The model under review builds one solid part; all positions refer to its coordinate system, in mm. Face numbers are marked on the shaded views. A direction names the side the tool comes from. Coordinates: 2 decimals unless noted, no trailing zeros. Write each loop counter-clockwise with the first axis right and the second up, starting at its lowest first coordinate (ties: lowest second). Pieces come first, ordered by that corner, then holes. Notation, with made-up numbers: (-36.75, 51.25) -> (19.25, 51.25) arc R15 ccw to (19.25, 57.25) -> close; hole circle Ø5 at (-26.75, 48.5). An arc over 180 degrees is marked (long way). Write each question's results on one line, items separated by ' | '.
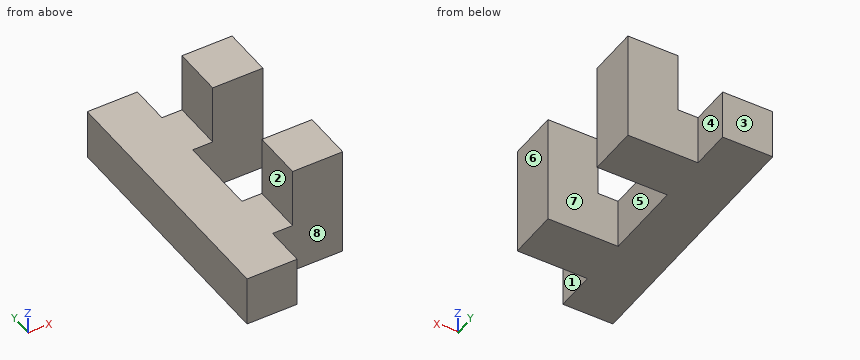
```python
from build123d import *

# Parameters (mm, degrees)
F1_DEPTH = 63.5
F2_W     = 63.5
F2_H     = 63.5
F3_DEPTH = 76.2


with BuildPart() as f1:
    # F0 (on Top) → F1 (new body)
    with BuildSketch(Plane.XY):
        Polygon((63.5, 0), (0, 0), (0, -330.2), (63.5, -330.2), (63.5, -279.4), (152.4, -279.4), (152.4, -215.9), (63.5, -215.9), (63.5, -114.3), (152.4, -114.3), (152.4, -50.8), (63.5, -50.8), align=None)
    extrude(amount=F1_DEPTH)

    # F2 (on face) → F3 (join)
    with BuildSketch(Plane.XY.offset(63.5)):
        with Locations((120.65, -82.55)):
            Rectangle(F2_W, F2_H)
        with Locations((120.65, -247.65)):
            Rectangle(F2_W, F2_H)
    extrude(amount=F3_DEPTH)


solid = f1.part
```
Q1. For line 1 (Y direction, x = 109, z = 94.5); line 2 (X direction, y = -224.5, z = 122); line 3 (X direction, y = -115, z = 59), list the stretches that pass through material, from the lowest coordinate up. Write a range as from..to.
Solution:
line 1: -279.4..-215.9, -114.3..-50.8 | line 2: 88.9..152.4 | line 3: 0..63.5
Q2. Add section B-B (x = 73). Write out the cut boundary in (y, z).
Solution:
outline: (-279.4, 0) -> (-215.9, 0) -> (-215.9, 63.5) -> (-279.4, 63.5) -> close; (-114.3, 0) -> (-50.8, 0) -> (-50.8, 63.5) -> (-114.3, 63.5) -> close
Q3. Machinability: for the marked faces 1, 2, 3, 4 and 5, which of the approach directions +Z, -Z, +X, -X, +Y, -Y give a long, thin tool a straight path to every point of the face, cutting with its end or side? Answer none if there is none.
Solution:
face 1: +Z, -Z, +X, -Y | face 2: +Z, -X, +Y, -Y | face 3: +Z, -Z, +X, -X, +Y | face 4: +Z, -Z, +X, +Y | face 5: +Z, -Z, +X
Q4. Clearance check with flat-ended pins moving along their axes: P1, Ø15, axis at y = -38, z = 18.5, coming from the +X side; P2, Ø3, axis at y = -97, z = 79.5, coming from the -X side; P3, Ø1.5, axis at x = 35.5, y = -232, coming from the +Z side; P4, Ø5, axis at y = -71.5, z = 17.5, coming from the -X side. State where each tip first meets the part, or that it passes through.
Solution:
P1: x = 63.5 | P2: x = 88.9 | P3: z = 63.5 | P4: x = 0
Q5. Draft analysis for pull direction Y (two halves, no side actions). For the marked faces 6, 7 and 8, state which applies: pulls with the +Y half, pulls with the -Y half, needs draft (parallel to the pull), parting line crosses it, or undercut.
Solution:
face 6: needs draft | face 7: undercut | face 8: pulls with the -Y half
Q6. Add section C-C (z = 55.5). Write out the cut boundary in (x, y).
Solution:
outline: (0, -330.2) -> (63.5, -330.2) -> (63.5, -279.4) -> (152.4, -279.4) -> (152.4, -215.9) -> (63.5, -215.9) -> (63.5, -114.3) -> (152.4, -114.3) -> (152.4, -50.8) -> (63.5, -50.8) -> (63.5, 0) -> (0, 0) -> close
Q7. Add section A-A (z = 126.5). Write out the cut boundary in (x, y), plus the area to 3 significant figures.
Solution:
outline: (88.9, -279.4) -> (152.4, -279.4) -> (152.4, -215.9) -> (88.9, -215.9) -> close; (88.9, -114.3) -> (152.4, -114.3) -> (152.4, -50.8) -> (88.9, -50.8) -> close | area: 8,060 mm²
Q8. Add section D-D (y = -100). Write out the cut boundary in (x, z), plus the area to 3 significant figures.
Solution:
outline: (0, 0) -> (152.4, 0) -> (152.4, 139.7) -> (88.9, 139.7) -> (88.9, 63.5) -> (0, 63.5) -> close | area: 14,500 mm²
